Read the model definition and answer for the solid it produces. Units are mm, in the model's axes. A direction names the side the tool comes from. Coordinates: 2 decimals unless noted, no trailing zeros. Order: outer loops, then holes, each group sorted by start corner. A loop starts at its lowest first (then second) coordinate and runs counter-clockwise, first axis right, second up. Notation, with made-up numbers: (35.5, 64.25) -> (53.5, 64.25) arc R33 ccw to (53.5, 93.25) -> close; hole circle Ø10 at (40.25, 73). An arc over 180 degrees is marked (long way). Answer as a JSON object with one key per item and string values. Group by question number.
1) A tool of negligible diameter and unlimited length cuts with its end or side. For faces 4 (the flat face through (100, 51, 2)), 5 (the flat face through (0, 101, 2)), from which of +Z, -Z, +X, -X, +Y, -Y can it reach the whole face along a straight path? Write none if from no direction.
2) Determine the mould class of faces 1 (the flat face through (49.256, 107.349, 1.232)), 2 (the flat face through (-11.457, 31.087, 2.465)), 3 (the flat face through (49.3, 107.403, 3.732)) for opening direction Z: released by +Z, released by -Z, zero draft, split by the parting line, or undercut.
3) Section B-B on z = 4.2 is taken. Determine the outline of the cut face in (x, y).
4) Given pin 1 (3 mm diameter, centred on y = 118.5, z = 2, fed in from +X); pin 2 (2.5 mm diameter, centred on y = 113, z = 2, fed in from -X); pin 3 (1 mm diameter, centred on y = 37.5, z = 4, fed in from -X), each flat-ended and moving along its own axis, determine where each tip first touches the part or whether it passes through.
5) Consider L1, parallel to X at y = 59.5, z = 4.05; L2, parallel to X at y = 25.5, z = 2.5. Determine where each line is inside the solid, lowest interval first.
from build123d import *

# Parameters (mm, degrees)
BOSS_EXTRUDE1_DEPTH = 5
CHAMFER6_SIZE       = 5
CHAMFER6_SIZE2      = 2.5
CHAMFER7_SIZE2      = 5
CHAMFER7_SIZE       = 2.5
CHAMFER8_SIZE       = 2.5
CHAMFER8_SIZE2      = 25
CHAMFER9_SIZE       = 2.5
CHAMFER9_SIZE_2     = 25


# Some blends are built 0.0001 mm under size
with BuildPart() as part:
    # Sketch1 → Boss-Extrude1 (new body)
    with BuildSketch(Plane.XY):
        Polygon((-30, -6), (0, 0), (0, 54), align=None)
        Polygon((100, 20), (0, 0), (0, 150), (100, 70), align=None)
    extrude(amount=BOSS_EXTRUDE1_DEPTH)

    # Chamfer6
    chamfer6_edges = [part.edges().sort_by_distance(p)[0] for p in [
        (50, 110, 5),
    ]]
    chamfer6_side = [part.faces().sort_by_distance(p)[0] for p in [
        (37.795251311, 59.015726179, 5),
    ]]
    chamfer(chamfer6_edges, length=CHAMFER6_SIZE, length2=CHAMFER6_SIZE2, reference=chamfer6_side[0])

    # Chamfer7
    chamfer7_edges = [part.edges().sort_by_distance(p)[0] for p in [
        (50, 110, 0),
    ]]
    chamfer7_side = [part.faces().sort_by_distance(p)[0] for p in [
        (50, 110, 0.05),
    ]]
    chamfer(chamfer7_edges, length=CHAMFER7_SIZE - 0.0001, length2=CHAMFER7_SIZE2 - 0.0001, reference=chamfer7_side[0])  # a hair under: the kernel refuses the full size

    # Chamfer8
    chamfer8_edges = [part.edges().sort_by_distance(p)[0] for p in [
        (35, 7, 5),
    ]]
    chamfer8_side = [part.faces().sort_by_distance(p)[0] for p in [
        (35, 7, 2.5),
    ]]
    chamfer(chamfer8_edges, length=CHAMFER8_SIZE, length2=CHAMFER8_SIZE2, reference=chamfer8_side[0])

    # Chamfer9
    # the kernel refuses this chamfer: 25, 2.5 mm, written as the material it takes off along each edge
    with BuildSketch(Plane(origin=(-93.726044684, -18.745208937, 0), x_dir=(0.07010860495922276, -0.3505430247961141, 0.933918824779468), z_dir=(0.9805806756909202, 0.19611613513818388, 0))) as chamfer9_piece_1:
        Polygon((CHAMFER9_SIZE * 0.933918824779, -CHAMFER9_SIZE * 0.357485144758), (-CHAMFER9_SIZE_2 * 0.357485144758, -CHAMFER9_SIZE_2 * 0.933918824779), (0, 0), align=None)
    extrude(amount=262.550645501, mode=Mode.SUBTRACT)


solid = part.part
Worked answers:
{
 "1": {"face 4": "+Z, -Z, +X, +Y, -Y", "face 5": "+Z, -Z, -X, +Y"},
 "2": {"face 1": "released by -Z", "face 2": "zero draft", "face 3": "released by +Z"},
 "3": {"outline": "(-20.37, 13.26) -> (100, 37.34) -> (100, 65.65) -> (0, 145.65) -> (0, 54) -> close"},
 "4": {"pin 1": "stops at x = 41.14", "pin 2": "stops at x = 0", "pin 3": "stops at x = -8.5"},
 "5": {"L1": "x = 0 to 100", "L2": "x = -14.25 to 100"}
}
